The listing builds one solid part. Answer for the finished solid, in the listing's coordinates (mm). A direction names the side the tool comes from. Round coordinates to 2 decimals unless told otherwise and drop trailing zeros. Write each loop counter-clockwise with the first axis right and the second up, starting at its lowest first coordinate (ties: lowest second). Pieces come first, ordered by that corner, then holes.
from build123d import *

# Parameters (mm, degrees)
ESQUISSE1_R             = 7.5
BASE_EXTRUSION_DEPTH    = 16
ESQUISSE2_R             = 13
ENL_V_MAT_EXTRU_2_DEPTH = 14


with BuildPart() as part:
    # Esquisse1 → Base-Extrusion (new body)
    with BuildSketch(Plane.XY):
        with BuildLine():
            ThreePointArc((25.740280008, -52.821275395), (-20, -34.641016151), (-58.614706356, -4.118901311))
            ThreePointArc((-58.614706356, -4.118901311), (-60.251834367, 0), (-58.614706356, 4.118901311))
            ThreePointArc((-58.614706356, 4.118901311), (-20, 34.641016151), (25.740280008, 52.821275395))
            ThreePointArc((25.740280008, 52.821275395), (30.125917184, 52.179619187), (32.874426349, 48.702374085))
            ThreePointArc((32.874426349, 48.702374085), (40, 0), (32.874426349, -48.702374085))
            ThreePointArc((32.874426349, -48.702374085), (30.125917184, -52.179619187), (25.740280008, -52.821275395))
        make_face()
        Circle(ESQUISSE1_R, mode=Mode.SUBTRACT)
    extrude(amount=BASE_EXTRUSION_DEPTH)

    # Esquisse2 → Enlèv. mat.-Extru.2 (cut)
    with BuildSketch(Plane.XY):
        Circle(ESQUISSE2_R)
    extrude(amount=ENL_V_MAT_EXTRU_2_DEPTH, mode=Mode.SUBTRACT)


solid = part.part
1. Section B-B on y = 0 is taken. Determine the outline of the cut face in (x, z), plus the area to 3 significant figures.
Geometry says:
outline: (-60.25, 0) - (-13, 0) - (-13, 14) - (-7.5, 14) - (-7.5, 16) - (-60.25, 16) - close; (7.5, 14) - (13, 14) - (13, 0) - (40, 0) - (40, 16) - (7.5, 16) - close
area: 1,210 mm2
2. Section D-D on x = -48.5 is taken. Determine the outline of the cut face in (y, z).
Geometry says:
outline: (-13.98, 0) - (13.98, 0) - (13.98, 16) - (-13.98, 16) - close
3. Straight lines are drawn through the part: line 1 along X through (y, z) = (0, 15.3); line 2 along Y through (x, z) = (0, 15.55); line 3 along Y through (x, z) = (0, 9.75). For each, find the intervals that lie inside material, in ascending order.
Geometry says:
line 1: x = -60.25 to -7.5, 7.5 to 40
line 2: y = -44.5 to -7.5, 7.5 to 44.5
line 3: y = -44.5 to -13, 13 to 44.5
4. For a pull along X with two mould halves and no side action, classify faces 1 (the face through (-9, 13, 0)), 2 (the face through (-10.316, -7.91, 6.902)), 3 (the face through (-19.4, -34.986, 7.888)) as released by +X, released by -X, zero draft, split by the parting line, or undercut.
Geometry says:
face 1: zero draft
face 2: undercut
face 3: released by -X
5. A tool of negligible diameter and unlimited length cuts with its end or side. For faces 4 (the face through (-9, 1, 16)), 5 (the face through (6, -6, 14)), from which of +Z, -Z, +X, -X, +Y, -Y can it reach the whole face along a straight path? Write none if from no direction.
Geometry says:
face 4: +Z, +X, -X, +Y, -Y
face 5: -Z
6. Section A-A on z = 10 is taken. Determine the outline of the cut face in (x, y), plus the area to 3 significant figures.
Geometry says:
outline: (-58.61, -4.12) arc R170 ccw to (25.74, -52.82) arc R6 ccw to (32.87, -48.7) arc R170 ccw to (32.87, 48.7) arc R6 ccw to (25.74, 52.82) arc R170 ccw to (-58.61, 4.12) arc R6 ccw to start; hole circle Ø26 at (0, 0)
area: 6,420 mm2
7. Given pin 1 (8 mm diameter, centred on y = 17.5, z = 7.5, fed in from -X); pin 2 (17 mm diameter, centred on x = 0, y = 0, fed in from -Z); pin 3 (3 mm diameter, centred on x = -43.5, z = 12, fed in from +Y), each flat-ended and moving along its own axis, determine where each tip first touches the part or whether it passes through.
Geometry says:
pin 1: stops at x = -49.03
pin 2: stops at z = 14
pin 3: stops at y = 19.52
8. Section C-C on x = 0 is taken. Determine the outline of the cut face in (y, z).
Geometry says:
outline: (-44.5, 0) - (-13, 0) - (-13, 14) - (-7.5, 14) - (-7.5, 16) - (-44.5, 16) - close; (7.5, 14) - (13, 14) - (13, 0) - (44.5, 0) - (44.5, 16) - (7.5, 16) - close
